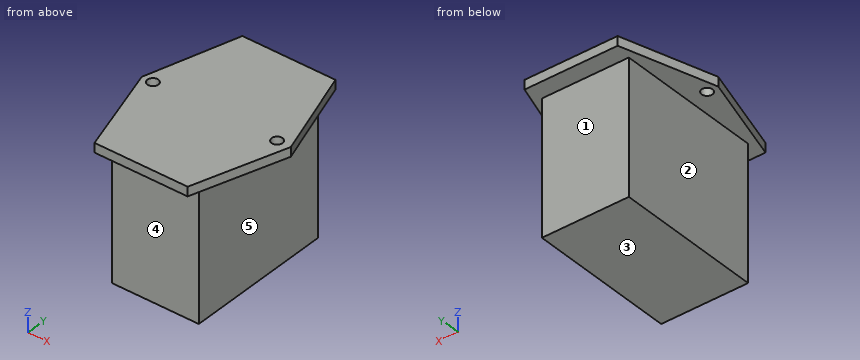
Autodesk Inventor part; units mm, degrees
ref_plane "YZ Plane" through (0, 0, 0) normal (1, 0, 0) x (0, 1, 0)
ref_plane "XZ Plane" through (0, 0, 0) normal (0, 1, 0) x (-1, 0, 0)
ref_plane "XY Plane" through (0, 0, 0) normal (0, 0, 1) x (1, 0, 0)
sketch "Skizze1" plane through (0, 0, 0) normal (0, 0, 1) x (1, 0, 0)
  line L0 (-14, -23.8) -> (-14, 23.8)
  line L1 (-14, 23.8) -> (14, 23.8)
  line L2 (14, 23.8) -> (14, -23.8)
  line L3 (14, -23.8) -> (-14, -23.8)
  line L4 (-14, -23.8) -> (14, 23.8) construction
  line L5 (-14, 23.8) -> (14, -23.8) construction
  point P0 (0, 0)
  dimension "d0" = 47.6
  dimension "d1" = 28
extrude "Extrusion1" add sketch "Skizze1" against normal blind 43
sketch "Skizze2" plane through (0, 0, 0) normal (0, 0, 1) x (1, 0, 0)
  line L0 (15, -29.5) -> (-15, -29.5)
  line L1 (-15, 29.5) -> (15, 29.5)
  line L2 (14, 23.8) -> (-14, 23.8)
  line L3 (-15, 29.5) -> (-23.5996, 0)
  line L4 (-23.5996, 0) -> (-15, -29.5)
  line L5 (15, -29.5) -> (24.4004, 0)
  line L6 (24.4004, 0) -> (15, 29.5)
  point P0 (0, 0)
  point P1 (0, 0)
  dimension "d4" = 5.7
  dimension "d15" = 59
  dimension "d16" = 48
  dimension "d17" = 30
extrude "Extrusion2" add sketch "Skizze2" along normal blind 3
sketch "Skizze3" plane through (0, 0, 3) normal (0, 0, 1) x (1, 0, 0)
  line L0 (15, 29.5) -> (-15, 29.5)
  line L1 (0, 29.5) -> (0, -29.5)
  line L2 (-15, -29.5) -> (15, -29.5)
  point P0 (0, 0)
  point P1 (-20, 0)
  point P2 (20, 0)
  dimension "d7" = 40
hole "Bohrung1" at (-20, 0, 3) at (20, 0, 3) direction (0, 0, -1) diameter 3.5 end through all
properties part number "Kaltstecker" material "Gummi, Silikon"
Geometry check sheet. Reference: the model listing, model coordinates, mm. Face numbers are marked on the shaded views. A direction names the side the tool comes from. Coordinates: 2 decimals unless noted, no trailing zeros. Write each loop counter-clockwise with the first axis right and the second up, starting at its lowest first coordinate (ties: lowest second). Pieces come first, ordered by that corner, then holes. Notation, with made-up numbers: (73.25, 62) -> (85.25, 62) arc R21 cw to (85.25, 88) -> close; hole circle Ø11 at (6.25, 65). An arc over 180 degrees is marked (long way). Use CSV: the item, a comma, the result in double quotes. Start each with the question number.
Item 1: Set-up check for the marked faces 1, 2, 3, 4 and 5: record each of +Z, -Z, +X, -X, +Y, -Y from which the full face is reachable in a straight line by a thin tool's end or side.
Item 2: Thickness scan on line 1 (X direction, y = 0, z = 1.55); line 2 (Y direction, x = 7, z = -36.5); line 3 (X direction, y = 2, z = -12). Record the ranges inside material, lowest first.
Item 3: Cross-section at D-D, the plane y = 5. Record the cut outline in (x, z), plus the area to 3 significant figures.
Item 4: Cross-section at C-C, the plane z = -36. Record the cut outline in (x, y).
Item 5: Depth check by flat-ended pin: pin 1 Ø22.5 at (x, z) = (-3.5, -21) entering from -Y; pin 2 Ø2 at (x, y) = (15.5, -15.5) entering from -Z; pin 3 Ø14 at (x, z) = (-1.5, -20) entering from +Y; pin 4 Ø2 at (x, y) = (-20, 0) entering from +Z. Enter the tip coordinate at first touch or a pass-through.
Item 6: Cross-section at A-A, the plane x = -20. Record the cut outline in (y, z).
Item 7: Cross-section at B-B, the plane x = 13. Record the cut outline in (y, z).
Answers:
1,face 1,"-Z, +X, -X, +Y"
1,face 2,"-Z, -X, +Y, -Y"
1,face 3,"-Z, +X, -X, +Y, -Y"
1,face 4,"-Z, +X, -X, -Y"
1,face 5,"-Z, +X, +Y, -Y"
2,line 1,"-23.6 to -21.75, -18.25 to 18.25, 21.75 to 24.4"
2,line 2,"-23.8 to 23.8"
2,line 3,"-14 to 14"
3,outline,"(-22.14, 0) -> (-14, 0) -> (-14, -43) -> (14, -43) -> (14, 0) -> (22.81, 0) -> (22.81, 3) -> (-22.14, 3) -> close"
3,area,"1,340 mm^2"
4,outline,"(-14, -23.8) -> (14, -23.8) -> (14, 23.8) -> (-14, 23.8) -> close"
5,pin 1,"y = -23.8"
5,pin 2,"z = 0"
5,pin 3,"y = 23.8"
5,pin 4,"through"
6,outline,"(-12.35, 0) -> (-1.75, 0) -> (-1.75, 3) -> (-12.35, 3) -> close; (1.75, 0) -> (12.35, 0) -> (12.35, 3) -> (1.75, 3) -> close"
7,outline,"(-29.5, 0) -> (-23.8, 0) -> (-23.8, -43) -> (23.8, -43) -> (23.8, 0) -> (29.5, 0) -> (29.5, 3) -> (-29.5, 3) -> close"
